For this review, take the finished solid that the model builds, in its own axes (mm). Face numbers are marked on the shaded views. A direction names the side the tool comes from. Give positions to 0.01 mm unless a question says otherwise; leave off trailing zeros. Write each loop counter-clockwise with the first axis right and the second up, starting at its lowest first coordinate (ties: lowest second). Pieces come first, ordered by that corner, then holes. Notation, with made-up numbers: M -37,37 L 13,37 A10 ccw 13,44 Z; hole C 10.5,-33 d10. An arc over 180 degrees is marked long. Write item = value, one per line.
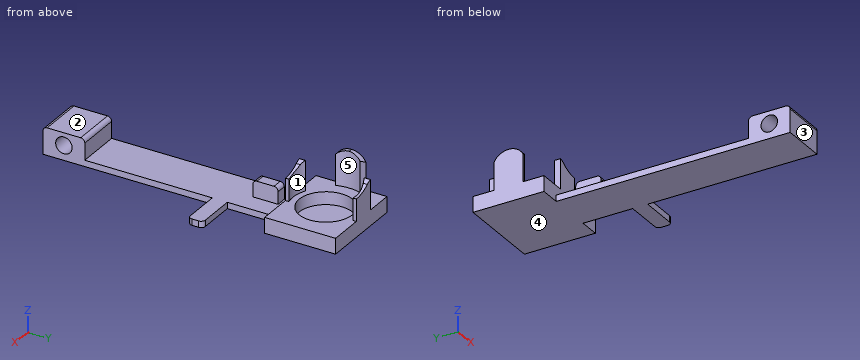
```python
from build123d import *

# Parameters (mm, degrees)
EXTRUDE_4_DEPTH          = 3.01
SKETCH_3_W               = 41.43
SKETCH_3_H               = 34.43
EXTRUDE_5_DEPTH          = 4.54
SKETCH_4_R               = 12.94
CUT_EXTRUDE_1_DEPTH      = 6.14
EXTRUDE_7_DEPTH          = 4.94
EXTRUDE_9_DEPTH          = 21.64
SKETCH_8_R               = 4
CUT_EXTRUDE_2_DEPTH      = 138.779016272
EXTRUDE_10_DEPTH         = 14.55
CUT_EXTRUDE_7_REACH      = 154.706
CUT_EXTRUDE_7_END_RADIUS = 16
EXTRUDE_11_DEPTH         = 17.51
CUT_EXTRUDE_8_REACH      = 144.669
CUT_EXTRUDE_8_END_RADIUS = 18.768238988


with BuildPart() as part:
    # 草图1 → 凸台-拉伸4 (new body)
    with BuildSketch(Plane.XY):
        with BuildLine():
            Line((10.82, -17.215), (10.82, -41.305))
            Line((10.82, -41.305), (28.54, -41.305))
            ThreePointArc((28.54, -41.305), (29.954213562, -41.890786438), (30.54, -43.305))
            Line((30.54, -43.305), (30.54, -46.575))
            ThreePointArc((30.54, -46.575), (29.954213562, -47.989213562), (28.54, -48.575))
            Line((28.54, -48.575), (10.82, -48.575))
            Line((10.82, -48.575), (10.82, -130.765))
            Line((10.82, -130.765), (-10.82, -130.765))
            Line((-10.82, -130.765), (-10.82, -17.215))
            Line((-10.82, -17.215), (-20.715, -17.215))
            Line((-20.715, -17.215), (-20.715, 17.215))
            Line((-20.715, 17.215), (20.715, 17.215))
            Line((20.715, 17.215), (20.715, -17.215))
            Line((20.715, -17.215), (10.82, -17.215))
        make_face()
    extrude(amount=EXTRUDE_4_DEPTH)

    # 草图3 → 凸台-拉伸5 (add)
    with BuildSketch(Plane.XY.offset(3.01)):
        Rectangle(SKETCH_3_W, SKETCH_3_H)
    extrude(amount=EXTRUDE_5_DEPTH)

    # 草图4 → 切除-拉伸1 (cut)
    with BuildSketch(Plane.XY.offset(7.55)):
        Circle(SKETCH_4_R)
    extrude(amount=-CUT_EXTRUDE_1_DEPTH, mode=Mode.SUBTRACT)

    # 草图6 → 凸台-拉伸7 (add)
    with BuildSketch(Plane.ZY.offset(3.55)):
        with BuildLine():
            Line((3.01, -22.315), (9.02, -22.315))
            ThreePointArc((9.02, -22.315), (10.434213562, -22.900786438), (11.02, -24.315))
            Line((11.02, -24.315), (11.02, -32.585))
            ThreePointArc((11.02, -32.585), (10.434213562, -33.999213562), (9.02, -34.585))
            Line((9.02, -34.585), (3.01, -34.585))
            Line((3.01, -34.585), (3.01, -22.315))
        make_face()
    extrude(amount=-EXTRUDE_7_DEPTH)

    # 草图7 → 凸台-拉伸9 (add)
    with BuildSketch(Plane.ZY.offset(10.82)):
        with BuildLine():
            Line((3.01, -130.765), (11.15, -130.765))
            ThreePointArc((11.15, -130.765), (12.564213562, -130.179213562), (13.15, -128.765))
            Line((13.15, -128.765), (13.15, -112.485))
            ThreePointArc((13.15, -112.485), (12.564213562, -111.070786438), (11.15, -110.485))
            Line((11.15, -110.485), (3.01, -110.485))
            Line((3.01, -110.485), (3.01, -130.765))
        make_face()
    extrude(amount=-EXTRUDE_9_DEPTH)

    # 草图8 → 切除-拉伸2 (cut, through all)
    with BuildSketch(Plane.ZY.offset(10.82)):
        with Locations((7.15, -120.625)):
            Circle(SKETCH_8_R)
    extrude(amount=-CUT_EXTRUDE_2_DEPTH, mode=Mode.SUBTRACT)

    # 草图9 → 凸台-拉伸10 (add)
    with BuildSketch(Plane.XY.offset(7.55)):
        with BuildLine():
            Line((3.994247308, 17.215), (-7.290402008, 17.215))
            Line((-7.290402008, 17.215), (-7.290402008, 14.242543262))
            ThreePointArc((-7.290402008, 14.242543262), (-1.762762206, 15.902599454), (3.994247308, 15.493417584))
            Line((3.994247308, 15.493417584), (3.994247308, 17.215))
        make_face()
    extrude_10 = extrude(amount=EXTRUDE_10_DEPTH)

    # 切除-拉伸7: up to this cylinder (the profile starts outside it)
    cut_extrude_7_end = Plane(origin=(0, 0, 20.532167), z_dir=(0, 0, -1)) * Cylinder(CUT_EXTRUDE_7_END_RADIUS, 342.412, mode=Mode.PRIVATE)
    # 草图10 → 切除-拉伸7 (cut, up to the surface)
    with BuildSketch(Plane(origin=(0, 17.215, 0), x_dir=(1, 0, 0), z_dir=(0, 1, 0)), mode=Mode.PRIVATE) as cut_extrude_7_sk1:
        with BuildLine():
            Line((3.994247308, -21.947856721), (3.994247308, -18.232150221))
            ThreePointArc((3.994247308, -18.232150221), (-0.624975177, -18.880311606), (-4.799480887, -20.961376627))
            ThreePointArc((-4.799480887, -20.961376627), (-5.989188818, -21.652656126), (-7.290402008, -22.1))
            Line((-7.290402008, -22.1), (3.994247308, -22.1))
            Line((3.994247308, -22.1), (3.994247308, -21.947856721))
        make_face()
    cut_extrude_7_tool1 = extrude(cut_extrude_7_sk1.sketch, amount=-CUT_EXTRUDE_7_REACH, mode=Mode.PRIVATE) - cut_extrude_7_end
    cut_extrude_7 = cut_extrude_7_tool1.solids().sort_by_distance((-0.002076, 17.215, 20.532167))[0]
    add(cut_extrude_7, mode=Mode.SUBTRACT)

    # 镜向1: 凸台-拉伸10, 切除-拉伸7 across plane
    add(extrude_10.mirror(Plane(origin=(0, 0, 0), x_dir=(0, 0, 1), z_dir=(0, -1, 0))))
    add(cut_extrude_7.mirror(Plane(origin=(0, 0, 0), x_dir=(0, 0, 1), z_dir=(0, -1, 0))), mode=Mode.SUBTRACT)

    # 草图12 → 凸台-拉伸11 (add)
    with BuildSketch(Plane.XY.offset(7.55)):
        with BuildLine():
            Line((-17.802400725, 5.943174502), (-20.715, 7.09508926))
            Line((-20.715, 7.09508926), (-20.715, -7.09508926))
            Line((-20.715, -7.09508926), (-17.802400725, -5.943174502))
            ThreePointArc((-17.802400725, -5.943174502), (-18.768238988, 0), (-17.802400725, 5.943174502))
        make_face()
    extrude(amount=EXTRUDE_11_DEPTH)

    # 切除-拉伸8: up to this cylinder (the profile starts outside it)
    cut_extrude_8_end = Plane(origin=(0, 0, 23.877666), z_dir=(0, 0, -1)) * Cylinder(CUT_EXTRUDE_8_END_RADIUS, 327.874477976, mode=Mode.PRIVATE)
    # 草图13 → 切除-拉伸8 (cut, up to the surface)
    with BuildSketch(Plane.ZY.offset(20.715), mode=Mode.PRIVATE) as cut_extrude_8_sk1:
        with BuildLine():
            ThreePointArc((25.06, 0), (23.920244617, -4.131873769), (20.823346631, -7.09508926))
            Line((20.823346631, -7.09508926), (25.06, -7.09508926))
            Line((25.06, -7.09508926), (25.06, 0))
        make_face()
    cut_extrude_8_tool1 = extrude(cut_extrude_8_sk1.sketch, amount=-CUT_EXTRUDE_8_REACH, mode=Mode.PRIVATE) - cut_extrude_8_end
    add(cut_extrude_8_tool1.solids().sort_by_distance((-20.715, -5.42758, 23.877666))[0], mode=Mode.SUBTRACT)
    # 草图13 → 切除-拉伸8 (cut, up to the surface)
    with BuildSketch(Plane.ZY.offset(20.715), mode=Mode.PRIVATE) as cut_extrude_8_sk2:
        with BuildLine():
            ThreePointArc((20.823346631, 7.09508926), (23.920244617, 4.131873769), (25.06, 0))
            Line((25.06, 0), (25.06, 7.09508926))
            Line((25.06, 7.09508926), (20.823346631, 7.09508926))
        make_face()
    cut_extrude_8_tool2 = extrude(cut_extrude_8_sk2.sketch, amount=-CUT_EXTRUDE_8_REACH, mode=Mode.PRIVATE) - cut_extrude_8_end
    add(cut_extrude_8_tool2.solids().sort_by_distance((-20.715, 5.42758, 23.877666))[0], mode=Mode.SUBTRACT)


solid = part.part
```
1. We need section C-C, the plane x = 0. Write out the cut boundary in (y, z) (3 decimals), then the cut area to 3 significant figures.
Responses:
outline = M -130.765,0 L 17.215,0 L 17.215,18.702 L 16,18.702 L 16,7.55 L 12.94,7.55 L 12.94,1.41 L -12.94,1.41 L -12.94,7.55 L -16,7.55 L -16,18.702 L -17.215,18.702 L -17.215,3.01 L -22.315,3.01 L -22.315,9.02 A2 ccw -24.315,11.02 L -32.585,11.02 A2 ccw -34.585,9.02 L -34.585,3.01 L -110.485,3.01 L -110.485,11.15 A2 ccw -112.485,13.15 L -128.765,13.15 A2 ccw -130.765,11.15 Z; hole C -120.625,7.15 d8
area = 720 mm2
2. We need section A-A, the plane z = 4.5. Write out the cut boundary in (x, y) (3 decimals), then the cut area to 3 significant figures.
Responses:
outline = M -20.715,-17.215 L 20.715,-17.215 L 20.715,17.215 L -20.715,17.215 Z; M -10.82,-130.765 L 10.82,-130.765 L 10.82,-123.621 L -10.82,-123.621 Z; M -10.82,-117.629 L 10.82,-117.629 L 10.82,-110.485 L -10.82,-110.485 Z; M -3.55,-34.585 L 1.39,-34.585 L 1.39,-22.315 L -3.55,-22.315 Z; hole C 0,0 d25.88
area = 1,270 mm2
3. We need section D-D, the plane y = -10. Write out the cut boundary in (x, z) (3 decimals), then the cut area to 3 significant figures.
Responses:
outline = M -20.715,0 L 20.715,0 L 20.715,7.55 L 8.212,7.55 L 8.212,1.41 L -8.212,1.41 L -8.212,7.55 L -20.715,7.55 Z
area = 212 mm2
4. Insertion check: P1, Ø3.5, axis at y = 16.5, z = 12, coming from the -X side; P2, Ø14.5, axis at y = -59, z = 6, coming from the -X side; P3, Ø8.5, axis at y = -1, z = 5, coming from the +X side (3 decimals). Each pin has a flat end and moves straight along its axis. Give the tip position at first contact, or say it passes through.
Responses:
P1 = -7.29
P2 = -10.82
P3 = 20.715
5. Machinability: for the marked faces 1, 2, 3, 4 and 5, which of the approach directions +Z, -Z, +X, -X, +Y, -Y give a long, thin tool a straight path to every point of the face, cutting with its end or side? Answer none if there is none.
Responses:
face_1 = +Z
face_2 = +Z, +X, -X, -Y
face_3 = +Z, -Z, +X, -X, -Y
face_4 = -Z, +X, -X, +Y, -Y
face_5 = +Z, +X
6. For line 1 along Y through (x, z) = (6, 7.15) (3 decimals); line 2 along Y through (x, z) = (-1, 4.25) (3 decimals); line 3 along Z through (x, y) = (3.5, 1), list the stretches that pass through material, from the lowest coordinate up. Write a range as from..to.
Responses:
line_1 = -130.765..-124.625, -116.625..-110.485, -17.215..-11.465, 11.465..17.215
line_2 = -130.765..-123.38, -117.87..-110.485, -34.585..-22.315, -17.215..-12.901, 12.901..17.215
line_3 = 0..1.41
7. We need section B-B, the plane x = 15.5. Write out the cut boundary in (y, z) (3 decimals), then the cut area to 3 significant figures.
Responses:
outline = M -48.575,0 L -41.305,0 L -41.305,3.01 L -48.575,3.01 Z; M -17.215,0 L 17.215,0 L 17.215,7.55 L -17.215,7.55 Z
area = 282 mm2
